Build history of the part. All positions in model axes, mm. A direction names the side the tool comes from. Coordinates: 2 decimals unless noted, no trailing zeros. Order: outer loops, then holes, each group sorted by start corner. A loop starts at its lowest first (then second) coordinate and runs counter-clockwise, first axis right, second up. Notation, with made-up numbers: (-6, 63) - (36, 63) arc R21 cw to (36, 80) - close; hole circle Ø7 at (78, 64.25). An arc over 180 degrees is marked (long way). Return JSON: item names as keys, results as strings.
from build123d import *

# Parameters (mm, degrees)
SKETCH1_W           = 52.5
SKETCH1_H           = 68
BOSS_EXTRUDE1_DEPTH = 46
CUT_EXTRUDE1_DEPTH  = 12.5
CUT_EXTRUDE2_DEPTH  = 23.5
CUT_EXTRUDE3_REACH  = 33.44
CUT_EXTRUDE4_REACH  = 23.389


with BuildPart() as part:
    # Sketch1 → Boss-Extrude1 (new body)
    with BuildSketch(Plane(origin=(0, 0, 0), x_dir=(1, 0, 0), z_dir=(0, 1, 0))):
        Rectangle(SKETCH1_W, SKETCH1_H)
    extrude(amount=BOSS_EXTRUDE1_DEPTH)

    # Sketch2 → Cut-Extrude1 (cut)
    with BuildSketch(Plane(origin=(0, 46, 0), x_dir=(1, 0, 0), z_dir=(0, 1, 0))):
        Polygon((26.25, 15), (10.25, 34), (-8.75, 34), (26.25, -4), align=None)
    extrude(amount=-CUT_EXTRUDE1_DEPTH, mode=Mode.SUBTRACT)

    # Sketch2_3 → Cut-Extrude2 (cut)
    with BuildSketch(Plane(origin=(0, 46, 0), x_dir=(1, 0, 0), z_dir=(0, 1, 0))):
        Polygon((26.25, -34), (26.25, -11), (-26.25, -34), align=None)
    extrude(amount=-CUT_EXTRUDE2_DEPTH, mode=Mode.SUBTRACT)

    # Sketch3 → Cut-Extrude3 (cut, up to next)
    with BuildSketch(Plane(origin=(8.911278514, 20.792983199, 20.340961825), x_dir=(0.956137046, -0.209388966, -0.204837032), z_dir=(0.292919697, 0.683479294, 0.668621048)), mode=Mode.PRIVATE) as cut_extrude3_sk1:
        Polygon((18.134138361, 7.870944216), (-36.774308303, -8.570238372), (18.134138361, -24.30435687), align=None)
    cut_extrude3_tool1 = extrude(cut_extrude3_sk1.sketch, amount=CUT_EXTRUDE3_REACH, mode=Mode.PRIVATE) & part.part
    add(cut_extrude3_tool1.solids().sort_by_distance((8.75, 15, 26.333333))[0], mode=Mode.SUBTRACT)

    # Sketch4 → Cut-Extrude4 (cut, up to next)
    with BuildSketch(Plane(origin=(-10.312326736, 34.813244868, 12.031047859), x_dir=(-0.962971205, -0.254816791, -0.088061685), z_dir=(0.269604261, -0.910153392, -0.314538305)), mode=Mode.PRIVATE) as cut_extrude4_sk1:
        Polygon((16.550519034, 47.160265119), (-37.968245086, 4.628461033), (16.550519034, -24.785895306), align=None)
    cut_extrude4_tool1 = extrude(cut_extrude4_sk1.sketch, amount=-CUT_EXTRUDE4_REACH, mode=Mode.PRIVATE) & part.part
    add(cut_extrude4_tool1.solids().sort_by_distance((-8.75, 38.166667, 3.666667))[0], mode=Mode.SUBTRACT)


solid = part.part
1. Cut at B-B on y = 43.5. Give the cut face in (x, z).
Check values:
{"outline": "(-26.25, -34) - (-8.75, -34) - (26.25, 4) - (26.25, 11) - (20.66, 13.45) - (-26.25, -26.77) - close; (10.25, -34) - (26.25, -34) - (26.25, -15) - close"}
2. Cut at A-A on x = -10.5. Give the cut face in (y, z), plus the area to 3 significant figures.
Check values:
{"outline": "(0, -34) - (46, -34) - (46, -20.5) - (29.55, 27.1) - (22.5, 27.1) - (15.75, 34) - (0, 34) - close", "area": "2,550 mm²"}
3. Cut at C-C on z = -11.5. Give the cut face in (x, y), plus the area to 3 significant figures.
Check values:
{"outline": "(-26.25, 0) - (26.25, 0) - (26.25, 33.5) - (11.97, 33.5) - (11.97, 46) - (0, 46) - (-26.25, 38.22) - close", "area": "2,130 mm²"}
4. Probe L1, parallel to Y at x = 8, z = -24.5; L2, parallel to Z at x = 18, y = 37.5; L3, parallel to Y at x = -3, z = 20. List the from-to ranges inside material, lowest first.
Check values:
{"L1": "0 to 33.5", "L2": "-34 to -24.8, -4.96 to 14.61", "L3": "0 to 34.23"}
5. Tool access for faces 1 (the flat face through (-6, 9, 34)), 2 (the flat face through (8.505, 39.838, -15.266)): list every direction of +Z, -Z, +X, -X, +Y, -Y with a clear straight run to the whole face (end or side of a thin tool).
Check values:
{"face 1": "+Z, +X, -X, +Y, -Y", "face 2": "+Y"}
6. Mould opens along X. For faces 3 (the flat face through (18.36, 39.84, -24.37)), 4 (the flat face through (0, 0, 0)), 5 (the flat face through (12.03, 29.19, 17.23)) say: pulls with the +X half, pulls with the -X half, needs draft (parallel to the pull), parting line crosses it, or undercut.
Check values:
{"face 3": "undercut", "face 4": "needs draft", "face 5": "pulls with the +X half"}
7. Cut at D-D on y = 18. Give the cut face in (x, z).
Check values:
{"outline": "(-26.25, -34) - (26.25, -34) - (26.25, 15.6) - (-15.75, 34) - (-26.25, 34) - close"}
8. Drop flat-ended pins along their axis: pin 1 (2 mm diameter, centred on y = 35, z = -13.5, fed in from +X); pin 2 (10 mm diameter, centred on y = 40.5, z = 0.5, fed in from +X); pin 3 (10 mm diameter, centred on x = 8.5, z = 22.5, fed in from +Y). Give the stop position or say it passes through.
Check values:
{"pin 1": "x = 11.05", "pin 2": "x = 26.25", "pin 3": "y = 38.94"}
